from build123d import *

# Parameters (mm, degrees)
F0_W      = 65.024
F0_H      = 84.074
F1_DEPTH  = 35.052
F2_W      = 5.588
F2_H      = 4.826
F3_DEPTH  = 127
F4_W      = 62.676213
F4_H      = 69.311896
F5_DEPTH  = 127
F7_DEPTH  = 127
F9_DEPTH  = 127
F11_DEPTH = 25.4
F12_R     = 8.001
F13_DEPTH = 65.025


with BuildPart() as f1:
    # F0 (on Right) → F1 (new body, symmetric)
    with BuildSketch(Plane.YZ):
        Rectangle(F0_W, F0_H)
    extrude(amount=F1_DEPTH, both=True)

    # F2 (on Front) → F3 (cut, symmetric)
    with BuildSketch(Plane.XZ):
        Polygon((-44.45, -3.937), (-44.45, -71.304262), (-12.7, -71.304262), (-12.7, -21.463), (-12.7, -16.637), (-12.7, -3.937), align=None)
        with Locations((-9.906, -19.05)):
            Rectangle(F2_W, F2_H)
        Polygon((44.45, -3.937), (12.7, -3.937), (12.7, -16.637), (12.7, -21.463), (12.7, -71.188014), (44.45, -71.188014), align=None)
        with Locations((9.906, -19.05)):
            Rectangle(F2_W, F2_H)
    extrude(amount=F3_DEPTH, both=True, mode=Mode.SUBTRACT)

    # F4 (on Right) → F5 (cut, symmetric)
    with BuildSketch(Plane.YZ):
        with Locations((38.450106, 27.670948)):
            Rectangle(F4_W, F4_H)
    extrude(amount=F5_DEPTH, both=True, mode=Mode.SUBTRACT)

    # F6 (on face) → F7 (cut, symmetric)
    with BuildSketch(Plane.YZ.offset(12.7)):
        Polygon((22.86, -6.985026), (32.512, -42.037), (51.482223, -29.319761), (47.049891, -1.715869), align=None)
    extrude(amount=F7_DEPTH, both=True, mode=Mode.SUBTRACT)

    # F8 (on Right) → F9 (cut, symmetric)
    with BuildSketch(Plane.YZ):
        with BuildLine():
            ThreePointArc((-27.939862, 15.211211), (-17.712772, 39.85918), (6.902644, 50.164375))
            Line((6.902644, 50.164375), (-42.650253, 55.479672))
            Line((-42.650253, 55.479672), (-50.782111, 15.211211))
            Line((-50.782111, 15.211211), (-27.939862, 15.211211))
        make_face()
    extrude(amount=F9_DEPTH, both=True, mode=Mode.SUBTRACT)

    # F10 (on face) → F11 (join)
    with BuildSketch(Plane.XZ.offset(32.512)):
        with BuildLine():
            Line((-12.7, 15.211211), (12.7, 15.211211))
            ThreePointArc((12.7, 15.211211), (0, 27.911211), (-12.7, 15.211211))
        make_face()
        with BuildLine():
            ThreePointArc((-12.7, 15.211211), (0, 2.511211), (12.7, 15.211211))
            Line((12.7, 15.211211), (-12.7, 15.211211))
        make_face()
    extrude(amount=-F11_DEPTH)

    # F12 (on face) → F13 (cut, through all)
    with BuildSketch(Plane.XZ.offset(32.512)):
        with Locations((0, 15.211211)):
            Circle(F12_R)
    extrude(amount=-F13_DEPTH, mode=Mode.SUBTRACT)


solid = f1.part
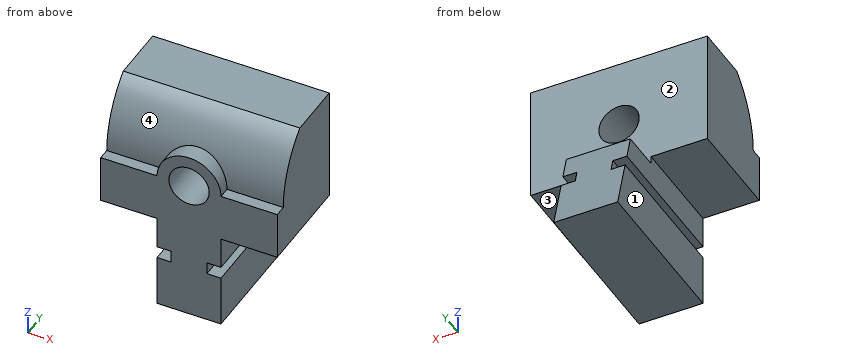
Here's how the part is built. I have some questions about the finished solid (model axes, mm). Face numbers are marked on the shaded views. A direction names the side the tool comes from. Coordinates: 2 decimals unless noted, no trailing zeros. Order: outer loops, then holes, each group sorted by start corner. A loop starts at its lowest first (then second) coordinate and runs counter-clockwise, first axis right, second up. Notation, with made-up numbers: M 81,-0.75 L 123,-0.75 A18 cw 123,9.25 Z; hole C 20,16 d11. An arc over 180 degrees is marked long. Answer as CSV lines item,"result".
Item 1: Imagine slicing it at C-C on y = 19.5. Write out the boundary of the cut face in (x, z) (3 decimals), plus the area to 3 significant figures.
Results found:
outline,"M -12.7,-42.037 L 12.7,-42.037 L 12.7,-21.463 L 7.112,-21.463 L 7.112,-16.637 L 12.7,-16.637 L 12.7,-6.985 L -12.7,-6.985 L -12.7,-16.637 L -7.112,-16.637 L -7.112,-21.463 L -12.7,-21.463 Z"
area,"836 mm2"
Item 2: Imagine slicing it at D-D on x = 15. Write out the boundary of the cut face in (y, z).
Results found:
outline,"M -32.51,-3.94 L 7.11,-3.94 L 7.11,42.04 L -15.33,42.04 A35.05 ccw -27.94,15.21 L -32.51,15.21 Z"
Item 3: For pin 1 (5.5 mm diameter, centred on y = 10.5, z = -20, fed in from -X); pin 2 (1.5 mm diameter, centred on x = -8.5, z = 4, fed in from +Y); pin 3 (11 mm diameter, centred on x = -25.5, y = -7.5, fed in from -Z); pin 4 (14.5 mm diameter, centred on x = 0, z = 15.21, fed in from +Y), each with a flat end and sliding along its axis, tell me the tip position at first contact or that it passes through.
Results found:
pin 1,"x = -12.7"
pin 2,"y = 7.11"
pin 3,"z = -3.94"
pin 4,"through"
Item 4: On a 3-axis mill with a long thin cutter (end or side, diameter ignored), from which of +Z, -Z, +X, -X, +Y, -Y can I reach the whole of each face in a straight line? I mean the marked faces 1, 2, 3 and 4. Say none if no direction works.
Results found:
face 1,"-Z, -X, +Y, -Y"
face 2,"+Z, +X, -X, +Y"
face 3,"-Z, +X, +Y, -Y"
face 4,"+Z, -Y"
Item 5: If I drill on line 1 (X direction, y = -28.5, z = 15); line 2 (Z direction, x = 0, y = -9.5); line 3 (X direction, y = -4.5, z = -21.5), over which ranges is the centre line in solid material (lowest first)?
Results found:
line 1,"-35.05 to -8, 8 to 35.05"
line 2,"-42.04 to 7.21, 23.21 to 42.04"
line 3,"-12.7 to 12.7"
Item 6: Imagine slicing it at A-A on y = 2.5. Write out the boundary of the cut face in (x, z), plus the area to 3 significant figures.
Results found:
outline,"M -35.05,-3.94 L -12.7,-3.94 L -12.7,-16.64 L -7.11,-16.64 L -7.11,-21.46 L -12.7,-21.46 L -12.7,-42.04 L 12.7,-42.04 L 12.7,-21.46 L 7.11,-21.46 L 7.11,-16.64 L 12.7,-16.64 L 12.7,-3.94 L 35.05,-3.94 L 35.05,42.04 L -35.05,42.04 Z; hole C 0,15.21 d16"
area,"3,940 mm2"
